```python
from build123d import *

# Parameters (mm, degrees)
F0_W     = 6.7386771552
F0_H     = 145.2977508307
F1_DEPTH = 9.652
F2_DEPTH = 3.302
F3_DEPTH = 48.768
F4_DEPTH = 17.526
F5_DEPTH = 16.256
F6_R     = 6.35
F7_R     = 6.35
F8_R     = 6.35


with BuildPart() as f1:
    # F0 (on Right) → F1 (new body)
    with BuildSketch(Plane.YZ):
        Rectangle(F0_W, F0_H)
    extrude(amount=F1_DEPTH)

    # F2 (add): a face of the model
    f2_faces = [f1.faces().sort_by_distance(p)[0] for p in [
        (4.826, -3.3693385776, 0),
    ]]
    extrude(f2_faces, amount=F2_DEPTH)

    # F3 (add): a face of the model
    f3_faces = [f1.faces().sort_by_distance(p)[0] for p in [
        (4.826, -1.651, -72.6488754153),
    ]]
    extrude(f3_faces, amount=F3_DEPTH)

    # F4 (add): a face of the model
    f4_faces = [f1.faces().sort_by_distance(p)[0] for p in [
        (9.652, -1.651, -24.384),
    ]]
    extrude(f4_faces, amount=F4_DEPTH)

    # F5 (add): a face of the model
    f5_faces = [f1.faces().sort_by_distance(p)[0] for p in [
        (13.589, -6.6713385776, -24.384),
    ]]
    extrude(f5_faces, amount=F5_DEPTH)

    # F6
    f6_edges = [f1.edges().sort_by_distance(p)[0] for p in [
        (27.178, -22.927339, -24.384),
    ]]
    fillet(f6_edges, radius=F6_R)

    # F7
    f7_edges = [f1.edges().sort_by_distance(p)[0] for p in [
        (27.178, 3.369339, -24.384),
    ]]
    fillet(f7_edges, radius=F7_R)

    # F8
    f8_edges = [f1.edges().sort_by_distance(p)[0] for p in [
        (0, -22.927339, -24.384),
        (0, 3.369339, -24.384),
    ]]
    fillet(f8_edges, radius=F8_R)


solid = f1.part
```
Input: part model. Units: mm. Frame: model coordinates. Give positions to 0.01 mm unless a question says otherwise; leave off trailing zeros. Write each loop counter-clockwise with the first axis right and the second up, starting at its lowest first coordinate (ties: lowest second). Pieces come first, ordered by that corner, then holes. Notation, with made-up numbers: (-2, -26) - (26, -26) arc R21 cw to (26, -5) - close; hole circle Ø11 at (36.5, -19.5). An arc over 180 degrees is marked (long way). Write item = value, one per line. Start each with the question number.
1) Cut plane A-A (z = -52). Return loops of the section in (x, y).
2) Material intervals for L1, parallel to X at y = -21, z = -79; L2, parallel to X at y = -1.75, z = -13; L3, parallel to Y at x = 25.5, z = 20, sorted ascending. Write a range as [from, to].
3) Cut plane B-B (y = -18.5). Return loops of the section in (x, z).
4) Cut plane C-C (x = 2). Return loops of the section in (y, z), and give its area (3 significant figures).
Answers follow:
q1.outline = (0, -16.58) arc R6.35 ccw to (6.35, -22.93) - (20.83, -22.93) arc R6.35 ccw to (27.18, -16.58) - (27.18, -2.98) arc R6.35 ccw to (20.83, 3.37) - (6.35, 3.37) arc R6.35 ccw to (0, -2.98) - close
q2.L1 = [1.79, 25.38]
q2.L2 = [0.12, 27.06]
q2.L3 = [-20.88, 1.32]
q3.outline = (0.3, -121.42) - (26.88, -121.42) - (26.88, 72.65) - (0.3, 72.65) - close
q4.outline = (-21.2, -121.42) - (1.65, -121.42) - (1.65, 72.65) - (-21.2, 72.65) - close
q4.area = 4,430 mm^2
